from build123d import *

# Parameters (mm, degrees)
CROQUIS1_R              = 1.5
SALIENTE_EXTRUIR1_DEPTH = 3
SALIENTE_EXTRUIR2_START = 3
CROQUIS2_W              = 5
CROQUIS2_H              = 18
SALIENTE_EXTRUIR2_DEPTH = 9
REDONDEO6_R             = 9
REDONDEO7_R             = 9
CORTAR_EXTRUIR1_REACH   = 47.338
CROQUIS3_R              = 2


with BuildPart() as part:
    # Croquis1 → Saliente-Extruir1 (new body)
    with BuildSketch(Plane.XY):
        with BuildLine():
            Line((-7.68763367, 13.798076923), (22.31236633, 13.798076923))
            ThreePointArc((22.31236633, 13.798076923), (25.847900236, 12.333610829), (27.31236633, 8.798076923))
            Line((27.31236633, 8.798076923), (27.31236633, -21.201923077))
            ThreePointArc((27.31236633, -21.201923077), (25.847900236, -24.737456983), (22.31236633, -26.201923077))
            Line((22.31236633, -26.201923077), (-7.68763367, -26.201923077))
            ThreePointArc((-7.68763367, -26.201923077), (-11.223167576, -24.737456983), (-12.68763367, -21.201923077))
            Line((-12.68763367, -21.201923077), (-12.68763367, 8.798076923))
            ThreePointArc((-12.68763367, 8.798076923), (-11.223167576, 12.333610829), (-7.68763367, 13.798076923))
        make_face()
        with Locations((7.31236633, 7.298076923)):
            Circle(CROQUIS1_R, mode=Mode.SUBTRACT)
        with Locations((7.31236633, -19.701923077)):
            Circle(CROQUIS1_R, mode=Mode.SUBTRACT)
    extrude(amount=SALIENTE_EXTRUIR1_DEPTH)

    # Croquis2 → Saliente-Extruir2 (add)
    with BuildSketch(Plane.XY.offset(SALIENTE_EXTRUIR2_START)):
        with Locations((-5.18763367, -6.201923077)):
            Rectangle(CROQUIS2_W, CROQUIS2_H)
        with Locations((19.81236633, -6.201923077)):
            Rectangle(CROQUIS2_W, CROQUIS2_H)
    extrude(amount=SALIENTE_EXTRUIR2_DEPTH)

    # Redondeo6
    redondeo6_edges = [part.edges().sort_by_distance(p)[0] for p in [
        (-5.18763367, 2.798076923, 12),
        (-5.18763367, -15.201923077, 12),
    ]]
    fillet(redondeo6_edges, radius=REDONDEO6_R - 0.0001)  # a hair under: the kernel refuses the full size

    # Redondeo7
    redondeo7_edges = [part.edges().sort_by_distance(p)[0] for p in [
        (19.81236633, -15.201923077, 12),
        (19.81236633, 2.798076923, 12),
    ]]
    fillet(redondeo7_edges, radius=REDONDEO7_R - 0.0001)  # a hair under: the kernel refuses the full size

    # Cortar-Extruir1: up to this face of the body (flat: up to its plane)
    cortar_extruir1_end = Plane(part.part.faces().sort_by_distance((22.31236633, -6.201923077, 6.819731779))[0])
    # Croquis3 → Cortar-Extruir1 (cut, up to the picked face)
    with BuildSketch(Plane.ZY.offset(7.68763367), mode=Mode.PRIVATE) as cortar_extruir1_sk1:
        with Locations((7.74625312, -6.201923077)):
            Circle(CROQUIS3_R)
    cortar_extruir1_tool1 = split(extrude(cortar_extruir1_sk1.sketch, amount=-CORTAR_EXTRUIR1_REACH, mode=Mode.PRIVATE), bisect_by=cortar_extruir1_end, keep=Keep.BOTH, mode=Mode.PRIVATE)
    add(cortar_extruir1_tool1.solids().sort_by(Axis((-7.687634, -6.201923, 7.746253), (1, 0, 0)))[0], mode=Mode.SUBTRACT)


solid = part.part
Geometry check sheet. Reference: the model listing, model coordinates, mm. A direction names the side the tool comes from. Give positions to 0.01 mm unless a question says otherwise; leave off trailing zeros. Loops run counter-clockwise (first coordinate to the right, second up) from the corner with the lowest first, then second, coordinate; pieces in that order, holes last. Notation, with made-up numbers: M 82,88.5 L 118,88.5 A23 cw 118,123.5 Z; hole C 30.25,53.5 d1. An arc over 180 degrees is marked long. Answer as a JSON object with one key per item and string values. Group by question number.
Item 1: Gauge pin test, flat ends, axial feed: pin 1 (3 mm diameter, centred on x = 4.5, y = -16, fed in from +Z); pin 2 (5 mm diameter, centred on y = -6.2, z = 7.75, fed in from -X); pin 3 (12 mm diameter, centred on x = 3, y = -3, fed in from +Z). Record the tip position at first contact, or that the pin passes through.
Item 2: Material ranges on L1, parallel to X at y = -8, z = 4; L2, parallel to Z at x = 18.5, y = -16.5; L3, parallel to Y at x = -3, z = 8.25, recorded low to high.
Item 3: Sectioned sample at D-D on x = 13.5. Record the boundary of the cut face in (y, z).
Item 4: Sectioned sample at A-A on z = 8. Record the boundary of the cut face in (x, y), plus the area to 3 significant figures.
Item 5: Sectioned sample at B-B on y = -5. Record the boundary of the cut face in (x, z), plus the area to 3 significant figures.
Item 6: Access from +Z, -Z, +X, -X, +Y, -Y to the whole of each face (thin tool, end or side, straight path). Record for faces 1 (the flat face through (-2.688, -6, 5)), 2 (the flat face through (8, -26.202, 1)).
Item 7: Mould release check, pull along X, two halves, no side actions. Record for faces 3 (the flat face through (27.312, -6, 1)), 4 (the cylindrical face through (-5.223, -8.154, 7.313)), 5 (the cylindrical face through (8.698, -20.276, 1.479)): pulls with the +X half, pulls with the -X half, needs draft (parallel to the pull), parting line crosses it, or undercut.
Findings below:
{
 "1": {"pin 1": "z = 3", "pin 2": "x = -7.69", "pin 3": "z = 11.91"},
 "2": {"L1": "-7.69 to -2.69, 17.31 to 22.31", "L2": "0 to 3", "L3": "-13.51 to -8.14, -4.27 to 1.11"},
 "3": {"outline": "M -26.2,0 L 13.8,0 L 13.8,3 L -26.2,3 Z"},
 "4": {"outline": "M -7.69,-13.69 L -2.69,-13.69 L -2.69,-8.19 L -7.69,-8.19 Z; M -7.69,-4.22 L -2.69,-4.22 L -2.69,1.28 L -7.69,1.28 Z; M 17.31,-13.69 L 22.31,-13.69 L 22.31,-8.19 L 17.31,-8.19 Z; M 17.31,-4.22 L 22.31,-4.22 L 22.31,1.28 L 17.31,1.28 Z", "area": "110 mm2"},
 "5": {"outline": "M -12.69,0 L 27.31,0 L 27.31,3 L 22.31,3 L 22.31,6.15 L 17.31,6.15 L 17.31,3 L -2.69,3 L -2.69,6.15 L -7.69,6.15 L -7.69,3 L -12.69,3 Z; M -7.69,9.34 L -2.69,9.34 L -2.69,11.92 L -7.69,11.92 Z; M 17.31,9.34 L 22.31,9.34 L 22.31,11.92 L 17.31,11.92 Z", "area": "177 mm2"},
 "6": {"face 1": "+Z, +Y, -Y", "face 2": "+Z, -Z, +X, -X, -Y"},
 "7": {"face 3": "pulls with the +X half", "face 4": "needs draft", "face 5": "undercut"}
}
